Build history of the part. All positions in model axes, mm. A direction names the side the tool comes from. Round coordinates to 2 decimals unless told otherwise and drop trailing zeros. Order: outer loops, then holes, each group sorted by start corner. A loop starts at its lowest first (then second) coordinate and runs counter-clockwise, first axis right, second up. Notation, with made-up numbers: (-34.75, -15) -> (-17.75, -15) arc R13 ccw to (-17.75, 0) -> close; hole circle Ø1 at (-3.75, 3). An arc over 180 degrees is marked (long way). Use a Markdown table: item, result. Add a question column.
Item 1: Slice it at D-D, the plane x = -20.5. Give the cut face in (y, z), plus the area to 3 significant figures.
Item 2: Two-plate mould, pull along Y, no slides. Class faces 1 (the face through (-26.65, 9, 0)), 2 (the face through (21.014, 17.263, -2.4)), 3 (the face through (7, -21.4, 0)): released by +Y, released by -Y, zero draft, split by the parting line, or undercut.
Item 3: Slice it at B-B, the plane z = 6.25. Give the cut face in (x, y) (3 decimals).
Item 4: Probe L1, parallel to Y at x = -11, z = -14.5; L2, parallel to X at y = 19, z = 14; L3, parallel to Y at x = -25.5, z = -10. List the from-to ranges inside material, lowest first.
Item 5: 3-axis set-ups, long thin cutter, end or side, ignore diameter. For faces 4 (the face through (23.41, -17.2, 14.69)), 5 (the face through (-28.622, 8.653, 5.534)), 6 (the face through (0, 0, -16.85)), 7 (the face through (31.679, 8.653, 6.966)): which of +Z, -Z, +X, -X, +Y, -Y reach the whole face in a straight line?
Item 6: Slice it at A-A, the plane y = 3.2. Give the cut face in (x, z), plus the area to 3 significant figures.
Item 7: Pin check, flat tips, straight feed: pin 1 (4 mm diameter, centred on y = 9, z = -11.5, fed in from +X); pin 2 (1 mm diameter, centred on y = -13.5, z = -1.5, fed in from -X); pin 3 (3 mm diameter, centred on x = 21.5, y = 16.5, fed in from +Z). Stop position of each tip, or through.
Item 8: Slice it at C-C, the plane z = 14. Give the cut face in (x, y) (3 decimals).
from build123d import *

# Parameters (mm, degrees)
ESBO_O1_W                                            = 53.3
ESBO_O1_H                                            = 33.7
RESSALTO_EXTRUS_O1_DEPTH                             = 21.4
CORTE_EXTRUS_O1_DEPTH                                = 34.7
ESBO_O3_R                                            = 5.5
RESSALTO_EXTRUS_O2_DEPTH                             = 10.2
ESBO_O4_R                                            = 5.5
RESSALTO_EXTRUS_O3_DEPTH                             = 4
REBAIXO_PARA_PARAFUSO_DE_M_QUINA_COM_CAB_D           = 2.9
REBAIXO_PARA_PARAFUSO_DE_M_QUINA_COM_CAB_CBORE_D     = 5.6
REBAIXO_PARA_PARAFUSO_DE_M_QUINA_COM_CAB_CBORE_DEPTH = 4.39


with BuildPart() as part:
    # Esboço1 → Ressalto-extrusão1 (new body, symmetric)
    with BuildSketch(Plane(origin=(0, 0, 0), x_dir=(1, 0, 0), z_dir=(0, 1, 0))):
        Rectangle(ESBO_O1_W, ESBO_O1_H)
    extrude(amount=RESSALTO_EXTRUS_O1_DEPTH, both=True)

    # Esboço2 → Corte-extrusão1 (cut, through all)
    with BuildSketch(Plane.XY.offset(16.85)):
        Polygon((-26.65, -21.4), (-11.35, -21.4), (-26.65, -4.093353878), align=None)
    extrude(amount=-CORTE_EXTRUS_O1_DEPTH, mode=Mode.SUBTRACT)

    # Esboço3 → Ressalto-extrusão2 (add)
    with BuildSketch(Plane(origin=(26.65, 0, 0), x_dir=(0, 0, -1), z_dir=(1, 0, 0))):
        with Locations((-6.25, 3.2)):
            Circle(ESBO_O3_R)
    extrude(amount=RESSALTO_EXTRUS_O2_DEPTH)

    # Esboço4 → Ressalto-extrusão3 (add)
    with BuildSketch(Plane.ZY.offset(26.65)):
        with Locations((6.25, 3.2)):
            Circle(ESBO_O4_R)
    extrude(amount=RESSALTO_EXTRUS_O3_DEPTH)

    # Rebaixo para parafuso de máquina com cabeça panela de M31 (through all)
    with Locations(Plane.XY.offset(16.85)):
        with Locations((20.825, 15.825), (20.825, -16.125), (-11.125, -16.125)):
            CounterBoreHole(REBAIXO_PARA_PARAFUSO_DE_M_QUINA_COM_CAB_D / 2, REBAIXO_PARA_PARAFUSO_DE_M_QUINA_COM_CAB_CBORE_D / 2, REBAIXO_PARA_PARAFUSO_DE_M_QUINA_COM_CAB_CBORE_DEPTH)


solid = part.part
Check sheet entries:
| question | item | result |
|---|---|---|
| 1 | outline | (-11.05, -16.85) -> (21.4, -16.85) -> (21.4, 16.85) -> (-11.05, 16.85) -> close |
| 1 | area | 1,090 mm2 |
| 2 | face 1 | zero draft |
| 2 | face 2 | undercut |
| 2 | face 3 | released by -Y |
| 3 | outline | (-30.65, -2.3) -> (-26.65, -2.3) -> (-26.65, -4.093) -> (-11.35, -21.4) -> (26.65, -21.4) -> (26.65, -2.3) -> (36.85, -2.3) -> (36.85, 8.7) -> (26.65, 8.7) -> (26.65, 21.4) -> (-26.65, 21.4) -> (-26.65, 8.7) -> (-30.65, 8.7) -> close; hole circle Ø2.9 at (-11.125, -16.125); hole circle Ø2.9 at (20.825, -16.125); hole circle Ø2.9 at (20.825, 15.825) |
| 4 | L1 | -21.4 to -17.57, -14.68 to 21.4 |
| 4 | L2 | -26.65 to 26.65 |
| 4 | L3 | -5.39 to 21.4 |
| 5 | face 4 | +Z |
| 5 | face 5 | -X |
| 5 | face 6 | -Z, +X, -X, +Y, -Y |
| 5 | face 7 | +X |
| 6 | outline | (-30.65, 0.75) -> (-26.65, 0.75) -> (-26.65, -16.85) -> (26.65, -16.85) -> (26.65, 0.75) -> (36.85, 0.75) -> (36.85, 11.75) -> (26.65, 11.75) -> (26.65, 16.85) -> (-26.65, 16.85) -> (-26.65, 11.75) -> (-30.65, 11.75) -> close |
| 6 | area | 1,950 mm2 |
| 7 | pin 1 | x = 26.65 |
| 7 | pin 2 | x = -18.78 |
| 7 | pin 3 | z = 12.46 |
| 8 | outline | (-26.65, -4.093) -> (-11.35, -21.4) -> (26.65, -21.4) -> (26.65, 21.4) -> (-26.65, 21.4) -> close; hole circle Ø5.6 at (-11.125, -16.125); hole circle Ø5.6 at (20.825, -16.125); hole circle Ø5.6 at (20.825, 15.825) |
